```python
from build123d import *

# Parameters (mm, degrees)
PAD_DEPTH   = 30
FILLET_R    = 2
FILLET001_R = 2
FILLET002_R = 2
FILLET003_R = 2
FILLET004_R = 2
FILLET005_R = 2
FILLET006_R = 2


with BuildPart() as part:
    # Sketch → Pad (new body)
    with BuildSketch(Plane.XY):
        Polygon((45, 40), (45, 0), (0, 0), (0, 15), (5, 15), (5, 5), (40, 5), (40, 40), align=None)
    extrude(amount=PAD_DEPTH)

    # Fillet
    fillet_edges = [part.edges().sort_by_distance(p)[0] for p in [
        (0, 15, 15),
    ]]
    fillet(fillet_edges, radius=FILLET_R)

    # Fillet001
    fillet001_edges = [part.edges().sort_by_distance(p)[0] for p in [
        (5, 15, 15),
    ]]
    fillet(fillet001_edges, radius=FILLET001_R)

    # Fillet002
    fillet002_edges = [part.edges().sort_by_distance(p)[0] for p in [
        (0, 0, 15),
    ]]
    fillet(fillet002_edges, radius=FILLET002_R)

    # Fillet003
    fillet003_edges = [part.edges().sort_by_distance(p)[0] for p in [
        (22.5, 5, 30),
    ]]
    fillet(fillet003_edges, radius=FILLET003_R)

    # Fillet004
    fillet004_edges = [part.edges().sort_by_distance(p)[0] for p in [
        (22.5, 5, 0),
    ]]
    fillet(fillet004_edges, radius=FILLET004_R)

    # Fillet005
    fillet005_edges = [part.edges().sort_by_distance(p)[0] for p in [
        (5, 9, 30),
    ]]
    fillet(fillet005_edges, radius=FILLET005_R)

    # Fillet006
    fillet006_edges = [part.edges().sort_by_distance(p)[0] for p in [
        (0, 7.5, 0),
    ]]
    fillet(fillet006_edges, radius=FILLET006_R)


solid = part.part
```
Geometry check sheet. Reference: the model listing, model coordinates, mm. A direction names the side the tool comes from. Round coordinates to 2 decimals unless told otherwise and drop trailing zeros. Order: outer loops, then holes, each group sorted by start corner. A loop starts at its lowest first (then second) coordinate and runs counter-clockwise, first axis right, second up. Notation, with made-up numbers: M 4,-27 L 43,-27 A15 ccw 43,-16 Z; hole C 24,-26.75 d5. An arc over 180 degrees is marked long. Write item = value, one per line.
Q1. Section check B-B (y = 6). Enter the section's corners in (x, z), plus the area to 3 significant figures.
Answer block:
outline = M 0,2 A2 ccw 2,0 L 3,0 A2 ccw 5,2 L 5,28 A2 ccw 3,30 L 2,30 A2 ccw 0,28 Z; M 40,0 L 45,0 L 45,30 L 40,30 Z
area = 297 mm^2
Q2. Set-up check for faces 4 (the cylindrical face through (4.4, 14.43, 15.18)), 5 (the cylindrical face through (2.51, 14.43, 0.6)), 6 (the cylindrical face through (4.43, 9.04, 29.4)): record each of +Z, -Z, +X, -X, +Y, -Y from which the full face is reachable in a straight line by a thin tool's end or side.
Answer block:
face_4 = +Z, -Z, +Y
face_5 = -Z, -X, +Y
face_6 = +Z, +Y
Q3. Depth check by flat-ended pin: pin 1 Ø0.5 at (x, z) = (2.5, 13) entering from +Y; pin 2 Ø12 at (y, z) = (32.5, 19) entering from -X; pin 3 Ø13 at (x, z) = (18, 11) entering from +Y. Enter the tip coordinate at first touch or a pass-through.
Answer block:
pin_1 = 15
pin_2 = 40
pin_3 = 5
Q4. Release check for a two-part mould opening along X. For faces 1 (the cylindrical face through (21.76, 4.4, 0.57)), 2 (the cylindrical face through (0.57, 7.58, 0.6)), 3 (the cylindrical face through (23.2, 0.57, 29.4)) record: released by +X, released by -X, zero draft, split by the parting line, or undercut.
Answer block:
face_1 = undercut
face_2 = released by -X
face_3 = zero draft
Q5. Section check A-A (x = 18). Enter the section's corners in (y, z), plus the area to 3 significant figures.
Answer block:
outline = M 0,2 A2 ccw 2,0 L 3,0 A2 ccw 5,2 L 5,28 A2 ccw 3,30 L 2,30 A2 ccw 0,28 Z
area = 147 mm^2
Q6. Section check D-D (y = 25). Enter the section's corners in (x, z), plus the area to 3 significant figures.
Answer block:
outline = M 40,0 L 45,0 L 45,30 L 40,30 Z
area = 150 mm^2
Q7. Scan lines: line 1 (X direction, y = 9.5, z = 5); line 2 (X direction, y = 19.5, z = 24.5); line 3 (Y direction, x = 27, z = 9.75). Record each from-to range of solid material in increasing order.
Answer block:
line_1 = 0 to 5, 40 to 45
line_2 = 40 to 45
line_3 = 0 to 5
Q8. Section check C-C (z = 9.25). Enter the section's corners in (x, y), plus the area to 3 significant figures.
Answer block:
outline = M 0,2 A2 ccw 2,0 L 45,0 L 45,40 L 40,40 L 40,5 L 5,5 L 5,13 A2 ccw 3,15 L 2,15 A2 ccw 0,13 Z
area = 447 mm^2
